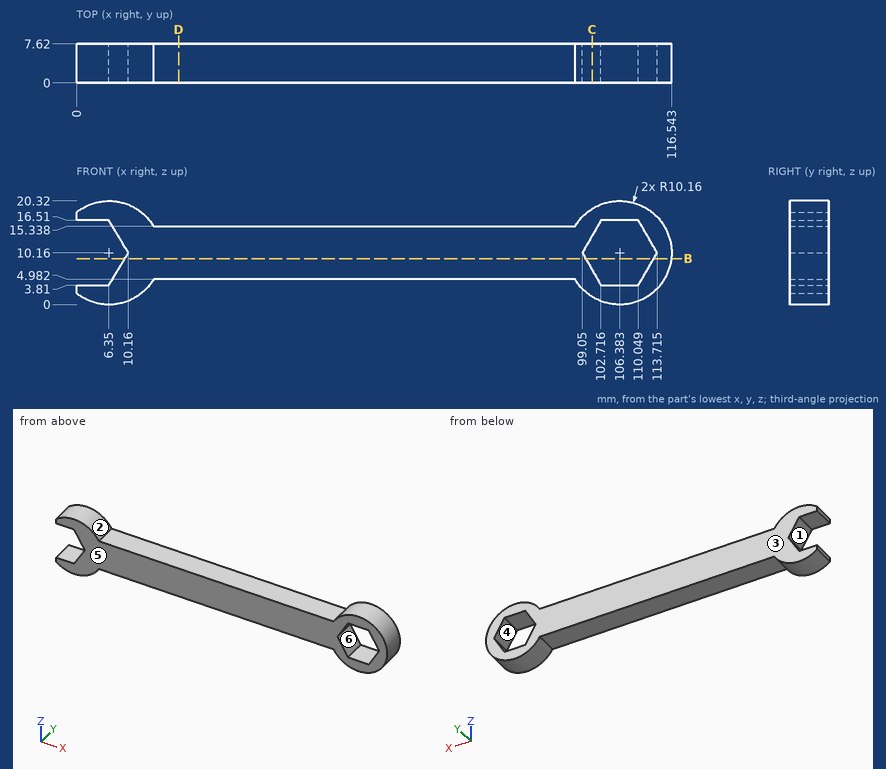
Can you work these out from the drawing? Everything is in mm from the part's minimum corner. A direction names the side the tool comes from. Coordinates: 2 decimals unless noted, no trailing zeros. Write each loop counter-clockwise with the first axis right and the second up, starting at its lowest first coordinate (ties: lowest second). Pieces come first, ordered by that corner, then holes. Notation, with made-up numbers: (-15, -8) -> (14, -8) arc R25 ccw to (14, 6) -> close; hole circle Ø2 at (-16.5, -37.5). An arc over 180 degrees is marked (long way). Write each question's results on one line, items separated by ' | '. Start each with the question number.
Q1. If I drill on probe 1 along Z at (x, y) = (40, 2); probe 2 along X at (y, z) = (3, 10.5) (1 decimal); probe 3 along X at (y, z) = (0.75, 2.25) (1 decimal), over which ranges is the centre line in solid material (lowest first)?
Q2. Imagine slicing it at B-B (z = 9). Write out the boundary of the cut face in (x, y) (1 decimal).
Q3. On a 3-axis mill with a long thin cutter (end or side, diameter ignored), from which of +Z, -Z, +X, -X, +Y, -Y can I reach the whole of each face in a straight line? I mean the marked faces 5 and 6. Say none if no direction works.
Q4. We'd pull the mould along Z, two halves only. Please class the marked faces 1, 2, 3 and 4: +Z half, -Z half, draft (parallel to the pull), parting line (faces both ways), or undercut.
Q5. I'm going to push flat-ended pins straight in: pin 1 (1 mm diameter, centred on x = 15, y = 6.5, fed in from -Z) (1 decimal); pin 2 (4 mm diameter, centred on x = 48.5, y = 1.5, fed in from -Z); pin 3 (1.9 mm diameter, centred on x = 3, y = 5.5, fed in from -Z). Where does each tip first touch, or does it pass through?
Q6. Imagine slicing it at C-C (x = 101). Write out the boundary of the cut face in (y, z).
Q7. Imagine slicing it at D-D (x = 20). Write out the boundary of the cut face in (y, z).
Taken from the geometry:
1) probe 1: z = 4.98 to 15.34 | probe 2: x = 10 to 99.2, 113.5 to 116.5 | probe 3: x = 0 to 12.7, 100 to 112.8
2) outline: (9.5, 0) -> (99.7, 0) -> (99.7, 7.6) -> (9.5, 7.6) -> close; (113, 0) -> (116.5, 0) -> (116.5, 7.6) -> (113, 7.6) -> close
3) face 5: +Z, -Z, +X, -X, -Y | face 6: +Y, -Y
4) face 1: undercut | face 2: +Z half | face 3: draft | face 4: undercut
5) pin 1: stops at z = 4.1 | pin 2: stops at z = 4.98 | pin 3: stops at z = 0.29
6) outline: (0, 1.54) -> (7.62, 1.54) -> (7.62, 6.78) -> (0, 6.78) -> close; (0, 13.54) -> (7.62, 13.54) -> (7.62, 18.78) -> (0, 18.78) -> close
7) outline: (0, 4.98) -> (7.62, 4.98) -> (7.62, 15.34) -> (0, 15.34) -> close
